Autodesk Inventor part; units mm, degrees
ref_plane "Arbeitsebene1" through (0, 0, 0.625) normal (0, 0, 1) x (1, 0, 0)
ref_plane "Arbeitsebene2" through (0, 0, 1.875) normal (0, 0, 1) x (1, 0, 0)
ref_plane "Arbeitsebene3" through (0, 0, 3.125) normal (0, 0, 1) x (1, 0, 0)
sketch "Skizze1" plane through (0, 0, 0) normal (0, 0, 1) x (1, 0, 0)
  circle A0 centre (0, 0) radius 4
extrude "Extrusion1" add sketch "Skizze1" along normal blind 180
ref_plane "Arbeitsebene1" through (0, 0, 0.625) normal (0, 0, 1) x (1, 0, 0)
sketch "Skizze2" plane through (0, 0, 0.625) normal (0, 0, 1) x (1, 0, 0)
  circle A0 centre (0, 0) radius 4
  circle A1 centre (0, 0) radius 3.25
extrude "Extrusion2" cut sketch "Skizze2" along normal mid plane 0.75
ref_plane "Arbeitsebene2" through (0, 0, 1.875) normal (0, 0, 1) x (1, 0, 0)
sketch "Skizze3" plane through (0, 0, 1.875) normal (0, 0, 1) x (1, 0, 0)
  circle A0 centre (0, 0) radius 4
  circle A1 centre (0, 0) radius 3.25
extrude "Extrusion3" cut sketch "Skizze3" along normal mid plane 0.75
ref_plane "Arbeitsebene3" through (0, 0, 3.125) normal (0, 0, 1) x (1, 0, 0)
sketch "Skizze4" plane through (0, 0, 3.125) normal (0, 0, 1) x (1, 0, 0)
  circle A0 centre (0, 0) radius 4
  circle A1 centre (0, 0) radius 3.25
extrude "Extrusion4" cut sketch "Skizze4" along normal mid plane 0.75
ref_plane "Arbeitsebene4" through (0, 0, 4.375) normal (0, 0, 1) x (1, 0, 0)
sketch "Skizze5" plane through (0, 0, 4.375) normal (0, 0, 1) x (1, 0, 0)
  circle A0 centre (0, 0) radius 4
  circle A1 centre (0, 0) radius 3.25
extrude "Extrusion5" cut sketch "Skizze5" along normal mid plane 0.75
ref_plane "Arbeitsebene5" through (0, 0, 5.625) normal (0, 0, 1) x (1, 0, 0)
sketch "Skizze6" plane through (0, 0, 5.625) normal (0, 0, 1) x (1, 0, 0)
  circle A0 centre (0, 0) radius 4
  circle A1 centre (0, 0) radius 3.25
extrude "Extrusion6" cut sketch "Skizze6" along normal mid plane 0.75
ref_plane "Arbeitsebene6" through (0, 0, 6.875) normal (0, 0, 1) x (1, 0, 0)
sketch "Skizze7" plane through (0, 0, 6.875) normal (0, 0, 1) x (1, 0, 0)
  circle A0 centre (0, 0) radius 4
  circle A1 centre (0, 0) radius 3.25
extrude "Extrusion7" cut sketch "Skizze7" along normal mid plane 0.75
ref_plane "Arbeitsebene7" through (0, 0, 8.125) normal (0, 0, 1) x (1, 0, 0)
sketch "Skizze8" plane through (0, 0, 8.125) normal (0, 0, 1) x (1, 0, 0)
  circle A0 centre (0, 0) radius 4
  circle A1 centre (0, 0) radius 3.25
extrude "Extrusion8" cut sketch "Skizze8" along normal mid plane 0.75
ref_plane "Arbeitsebene8" through (0, 0, 9.375) normal (0, 0, 1) x (1, 0, 0)
sketch "Skizze9" plane through (0, 0, 9.375) normal (0, 0, 1) x (1, 0, 0)
  circle A0 centre (0, 0) radius 4
  circle A1 centre (0, 0) radius 3.25
extrude "Extrusion9" cut sketch "Skizze9" along normal mid plane 0.75
ref_plane "Arbeitsebene9" through (0, 0, 10.625) normal (0, 0, 1) x (1, 0, 0)
sketch "Skizze10" plane through (0, 0, 10.625) normal (0, 0, 1) x (1, 0, 0)
  circle A0 centre (0, 0) radius 4
  circle A1 centre (0, 0) radius 3.25
extrude "Extrusion10" cut sketch "Skizze10" along normal mid plane 0.75
ref_plane "Arbeitsebene10" through (0, 0, 11.875) normal (0, 0, 1) x (1, 0, 0)
sketch "Skizze11" plane through (0, 0, 11.875) normal (0, 0, 1) x (1, 0, 0)
  circle A0 centre (0, 0) radius 4
  circle A1 centre (0, 0) radius 3.25
extrude "Extrusion11" cut sketch "Skizze11" along normal mid plane 0.75
ref_plane "Arbeitsebene11" through (0, 0, 13.125) normal (0, 0, 1) x (1, 0, 0)
sketch "Skizze12" plane through (0, 0, 13.125) normal (0, 0, 1) x (1, 0, 0)
  circle A0 centre (0, 0) radius 4
  circle A1 centre (0, 0) radius 3.25
extrude "Extrusion12" cut sketch "Skizze12" along normal mid plane 0.75
ref_plane "Arbeitsebene12" through (0, 0, 14.375) normal (0, 0, 1) x (1, 0, 0)
sketch "Skizze13" plane through (0, 0, 14.375) normal (0, 0, 1) x (1, 0, 0)
  circle A0 centre (0, 0) radius 4
  circle A1 centre (0, 0) radius 3.25
extrude "Extrusion13" cut sketch "Skizze13" along normal mid plane 0.75
ref_plane "Arbeitsebene13" through (0, 0, 15.625) normal (0, 0, 1) x (1, 0, 0)
sketch "Skizze14" plane through (0, 0, 15.625) normal (0, 0, 1) x (1, 0, 0)
  circle A0 centre (0, 0) radius 4
  circle A1 centre (0, 0) radius 3.25
extrude "Extrusion14" cut sketch "Skizze14" along normal mid plane 0.75
ref_plane "Arbeitsebene14" through (0, 0, 16.875) normal (0, 0, 1) x (1, 0, 0)
sketch "Skizze15" plane through (0, 0, 16.875) normal (0, 0, 1) x (1, 0, 0)
  circle A0 centre (0, 0) radius 4
  circle A1 centre (0, 0) radius 3.25
extrude "Extrusion15" cut sketch "Skizze15" along normal mid plane 0.75
ref_plane "Arbeitsebene15" through (0, 0, 18.125) normal (0, 0, 1) x (1, 0, 0)
sketch "Skizze16" plane through (0, 0, 18.125) normal (0, 0, 1) x (1, 0, 0)
  circle A0 centre (0, 0) radius 4
  circle A1 centre (0, 0) radius 3.25
extrude "Extrusion16" cut sketch "Skizze16" along normal mid plane 0.75
ref_plane "Arbeitsebene16" through (0, 0, 19.375) normal (0, 0, 1) x (1, 0, 0)
sketch "Skizze17" plane through (0, 0, 19.375) normal (0, 0, 1) x (1, 0, 0)
  circle A0 centre (0, 0) radius 4
  circle A1 centre (0, 0) radius 3.25
extrude "Extrusion17" cut sketch "Skizze17" along normal mid plane 0.75
ref_plane "Arbeitsebene17" through (0, 0, 20.625) normal (0, 0, 1) x (1, 0, 0)
sketch "Skizze18" plane through (0, 0, 20.625) normal (0, 0, 1) x (1, 0, 0)
  circle A0 centre (0, 0) radius 4
  circle A1 centre (0, 0) radius 3.25
extrude "Extrusion18" cut sketch "Skizze18" along normal mid plane 0.75
ref_plane "Arbeitsebene18" through (0, 0, 21.875) normal (0, 0, 1) x (1, 0, 0)
sketch "Skizze19" plane through (0, 0, 21.875) normal (0, 0, 1) x (1, 0, 0)
  circle A0 centre (0, 0) radius 4
  circle A1 centre (0, 0) radius 3.25
extrude "Extrusion19" cut sketch "Skizze19" along normal mid plane 0.75
ref_plane "Arbeitsebene19" through (0, 0, 23.125) normal (0, 0, 1) x (1, 0, 0)
sketch "Skizze20" plane through (0, 0, 23.125) normal (0, 0, 1) x (1, 0, 0)
  circle A0 centre (0, 0) radius 4
  circle A1 centre (0, 0) radius 3.25
extrude "Extrusion20" cut sketch "Skizze20" along normal mid plane 0.75
ref_plane "Arbeitsebene20" through (0, 0, 24.375) normal (0, 0, 1) x (1, 0, 0)
sketch "Skizze21" plane through (0, 0, 24.375) normal (0, 0, 1) x (1, 0, 0)
  circle A0 centre (0, 0) radius 4
  circle A1 centre (0, 0) radius 3.25
extrude "Extrusion21" cut sketch "Skizze21" along normal mid plane 0.75
ref_plane "Arbeitsebene21" through (0, 0, 25.625) normal (0, 0, 1) x (1, 0, 0)
sketch "Skizze22" plane through (0, 0, 25.625) normal (0, 0, 1) x (1, 0, 0)
  circle A0 centre (0, 0) radius 4
  circle A1 centre (0, 0) radius 3.25
extrude "Extrusion22" cut sketch "Skizze22" along normal mid plane 0.75
ref_plane "Arbeitsebene22" through (0, 0, 26.875) normal (0, 0, 1) x (1, 0, 0)
sketch "Skizze23" plane through (0, 0, 26.875) normal (0, 0, 1) x (1, 0, 0)
  circle A0 centre (0, 0) radius 4
  circle A1 centre (0, 0) radius 3.25
extrude "Extrusion23" cut sketch "Skizze23" along normal mid plane 0.75
ref_plane "Arbeitsebene23" through (0, 0, 28.125) normal (0, 0, 1) x (1, 0, 0)
sketch "Skizze24" plane through (0, 0, 28.125) normal (0, 0, 1) x (1, 0, 0)
  circle A0 centre (0, 0) radius 4
  circle A1 centre (0, 0) radius 3.25
extrude "Extrusion24" cut sketch "Skizze24" along normal mid plane 0.75
ref_plane "Arbeitsebene24" through (0, 0, 29.375) normal (0, 0, 1) x (1, 0, 0)
sketch "Skizze25" plane through (0, 0, 29.375) normal (0, 0, 1) x (1, 0, 0)
  circle A0 centre (0, 0) radius 4
  circle A1 centre (0, 0) radius 3.25
extrude "Extrusion25" cut sketch "Skizze25" along normal mid plane 0.75
ref_plane "Arbeitsebene25" through (0, 0, 30.625) normal (0, 0, 1) x (1, 0, 0)
sketch "Skizze26" plane through (0, 0, 30.625) normal (0, 0, 1) x (1, 0, 0)
  circle A0 centre (0, 0) radius 4
  circle A1 centre (0, 0) radius 3.25
extrude "Extrusion26" cut sketch "Skizze26" along normal mid plane 0.75
ref_plane "Arbeitsebene26" through (0, 0, 31.875) normal (0, 0, 1) x (1, 0, 0)
sketch "Skizze27" plane through (0, 0, 31.875) normal (0, 0, 1) x (1, 0, 0)
  circle A0 centre (0, 0) radius 4
  circle A1 centre (0, 0) radius 3.25
extrude "Extrusion27" cut sketch "Skizze27" along normal mid plane 0.75
ref_plane "Arbeitsebene27" through (0, 0, 33.125) normal (0, 0, 1) x (1, 0, 0)
sketch "Skizze28" plane through (0, 0, 33.125) normal (0, 0, 1) x (1, 0, 0)
  circle A0 centre (0, 0) radius 4
  circle A1 centre (0, 0) radius 3.25
extrude "Extrusion28" cut sketch "Skizze28" along normal mid plane 0.75
ref_plane "Arbeitsebene28" through (0, 0, 34.375) normal (0, 0, 1) x (1, 0, 0)
sketch "Skizze29" plane through (0, 0, 34.375) normal (0, 0, 1) x (1, 0, 0)
  circle A0 centre (0, 0) radius 4
  circle A1 centre (0, 0) radius 3.25
extrude "Extrusion29" cut sketch "Skizze29" along normal mid plane 0.75
ref_plane "Arbeitsebene29" through (0, 0, 35.625) normal (0, 0, 1) x (1, 0, 0)
sketch "Skizze30" plane through (0, 0, 35.625) normal (0, 0, 1) x (1, 0, 0)
  circle A0 centre (0, 0) radius 4
  circle A1 centre (0, 0) radius 3.25
extrude "Extrusion30" cut sketch "Skizze30" along normal mid plane 0.75
ref_plane "Arbeitsebene30" through (0, 0, 36.875) normal (0, 0, 1) x (1, 0, 0)
sketch "Skizze31" plane through (0, 0, 36.875) normal (0, 0, 1) x (1, 0, 0)
  circle A0 centre (0, 0) radius 4
  circle A1 centre (0, 0) radius 3.25
extrude "Extrusion31" cut sketch "Skizze31" along normal mid plane 0.75
properties part number "Gewindestange_M8"
Geometry check sheet. Reference: the model listing, model coordinates, mm. A direction names the side the tool comes from. Round coordinates to 2 decimals unless told otherwise and drop trailing zeros. Order: outer loops, then holes, each group sorted by start corner. A loop starts at its lowest first (then second) coordinate and runs counter-clockwise, first axis right, second up. Notation, with made-up numbers: (29.25, -24.75) - (47.25, -24.75) arc R25 ccw to (47.25, -0.75) - close; hole circle Ø3 at (-24.75, 87). An arc over 180 degrees is marked (long way). One line per question, with ' | ' between items. Start each with the question number.
(1) Access from +Z, -Z, +X, -X, +Y, -Y to the whole of each face (thin tool, end or side, straight path). Record for faces 3 (the cylindrical face through (-0.867, 3.905, 17.496)), 4 (the flat face through (-2, 3, 21)).
(2) Sectioned sample at A-A on z = 101. Record the cut outline in (x, y), and give its area (3 significant figures).
(3) Thickness scan on L1, parallel to X at y = 0.25, z = 81; L2, parallel to X at y = -3.25, z = 39; L3, parallel to Y at x = 1, z = 134.5. Record the ranges inside material, lowest first. Write a range as [from, to].
(4) Release check for a two-part mould opening along Z. For faces 1 (the flat face through (-2, 3, 6)), 2 (the cylindrical face through (-0.867, 3.905, 16.247)) record: released by +Z, released by -Z, zero draft, split by the parting line, or undercut.
Conclusion:
1) face 3: +Z, -Z | face 4: none
2) outline: circle Ø8 at (0, 0) | area: 50.3 mm2
3) L1: x = [-3.99, 3.99] | L2: x = [-2.33, 2.33] | L3: y = [-3.87, 3.87]
4) face 1: undercut | face 2: zero draft
